from build123d import *

# Parameters (mm, degrees)
BOSS_EXTRUDE1_DEPTH  = 1.5875
M4_CLEARANCE_HOLE1_D = 4.5
BOSS_EXTRUDE2_DEPTH  = 3.175
FILLET1_R            = 3.5
M3_CLEARANCE_HOLE1_D = 3.4
SKETCH8_R            = 2.15
CUT_EXTRUDE1_DEPTH   = 4.1750001
SKETCH9_R            = 2.75
SKETCH9_R_2          = 2.15
BOSS_EXTRUDE3_DEPTH  = 0.75
SKETCH10_R           = 3.5
CUT_EXTRUDE2_DEPTH   = 2.5


with BuildPart() as part:
    # Sketch2 → Boss-Extrude1 (new body, symmetric)
    with BuildSketch(Plane.XY):
        with BuildLine():
            ThreePointArc((-17.942568571, -13.649816766), (-25.009816766, -13.417431429), (-24.777431429, -6.350183234))
            add(Edge.make_bspline(
                [(-24.777431429, -6.350183234), (-20.441430485, -2.271315687), (-12.829947979, 2.196277878), (-6.501150321, 4.42663028), (0, 5.19112324), (6.501150321, 4.42663028), (12.829947979, 2.196277878), (20.441430485, -2.271315687), (24.777431429, -6.350183234)],
                knots=[0, 0, 0, 0.1875, 0.3125, 0.4375, 0.5625, 0.6875, 0.8125, 1, 1, 1], degree=2))
            ThreePointArc((24.777431429, -6.350183234), (25.009816766, -13.417431429), (17.942568571, -13.649816766))
            add(Edge.make_bspline(
                [(-17.942568571, -13.649816766), (-14.268569515, -10.228684313), (-8.530052021, -6.883777878), (-4.178849679, -5.36413028), (0, -4.87862324), (4.178849679, -5.36413028), (8.530052021, -6.883777878), (14.268569515, -10.228684313), (17.942568571, -13.649816766)],
                knots=[0, 0, 0, 0.1875, 0.3125, 0.4375, 0.5625, 0.6875, 0.8125, 1, 1, 1], degree=2))
        make_face()
    extrude(amount=BOSS_EXTRUDE1_DEPTH, both=True)

    # M4 Clearance Hole1 (through all)
    with Locations(Plane.XY.offset(1.5875)):
        with Locations((21.36, -10), (0, 0)):
            Hole(M4_CLEARANCE_HOLE1_D / 2)

    # Sketch5 → Boss-Extrude2 (add)
    with BuildSketch(Plane(origin=(0, 0, -1.5875), x_dir=(-1, 0, 0), z_dir=(0, 0, -1))):
        with BuildLine():
            ThreePointArc((13.518770817, -20.368950039), (17.11, -26.460179221), (23.201229183, -22.868950039))
            Line((23.201229183, -22.868950039), (26.201229183, -11.25))
            ThreePointArc((26.201229183, -11.25), (22.61, -5.158770817), (16.518770817, -8.75))
            Line((16.518770817, -8.75), (13.518770817, -20.368950039))
        make_face()
    extrude(amount=-BOSS_EXTRUDE2_DEPTH)

    # Fillet1
    fillet1_edges = [part.edges().sort_by_distance(p)[0] for p in [
        (-15.752223744, -11.718824048, 0.7937488),
    ]]
    fillet(fillet1_edges, radius=FILLET1_R)

    # M3 Clearance Hole1 (through all)
    with Locations(Plane(origin=(0, 0, -1.5875), x_dir=(-1, 0, 0), z_dir=(0, 0, -1))):
        with Locations((18.36, -21.618950039)):
            Hole(M3_CLEARANCE_HOLE1_D / 2)

    # Sketch8 → Cut-Extrude1 (cut, through all)
    with BuildSketch(Plane(origin=(0, 0, -1.5875), x_dir=(-1, 0, 0), z_dir=(0, 0, -1))):
        with Locations((21.36, -10)):
            Circle(SKETCH8_R)
    extrude(amount=-CUT_EXTRUDE1_DEPTH, mode=Mode.SUBTRACT)

    # Sketch9 → Boss-Extrude3 (add)
    with BuildSketch(Plane(origin=(0, 0, -1.5875), x_dir=(-1, 0, 0), z_dir=(0, 0, -1))):
        with Locations((21.36, -10)):
            Circle(SKETCH9_R)
        with Locations((21.36, -10)):
            Circle(SKETCH9_R_2, mode=Mode.SUBTRACT)
    extrude(amount=BOSS_EXTRUDE3_DEPTH)

    # Sketch10 → Cut-Extrude2 (cut)
    with BuildSketch(Plane.XY.offset(1.5875)):
        with Locations((21.36, -10)):
            Circle(SKETCH10_R)
    extrude(amount=-CUT_EXTRUDE2_DEPTH, mode=Mode.SUBTRACT)


solid = part.part
Read the model definition and answer for the solid it produces. Units are mm, in the model's axes. A direction names the side the tool comes from. Round coordinates to 2 decimals unless told otherwise and drop trailing zeros. Loops run counter-clockwise (first coordinate to the right, second up) from the corner with the lowest first, then second, coordinate; pieces in that order, holes last. Notation, with made-up numbers: (28.25, -18.5) - (44.25, -18.5) arc R12 cw to (44.25, -1.5) - close; hole circle Ø9 at (23.25, 6.25). An arc over 180 degrees is marked (long way). One line per question, with ' | ' between items. Start each with the question number.
Q1. Find the intervals of material crossed by L1, parallel to Y at x = 0, z = 0.65; L2, parallel to Y at x = -19.5, z = -1.4; L3, parallel to X at y = -11.5, z = -0.8, in increasing order.
Q2. For a pull along X with two mould halves and no side action, classify faces 4 (the cylindrical face through (-23.9, -11.05, -1.96)), 5 (the flat face through (-23, -12, -2.338)), 6 (the cylindrical face through (-18.73, -23.28, 0.02)) as +X half, -X half, draft (parallel to the pull), parting line (faces both ways), or undercut.
Q3. For faces 1 (the flat face through (-14.362, -17.105, -0.022)), 2 (the flat face through (24, -10, -0.913)), 3 (the flat face through (-8, -6, 1.588)), determine the directions among +Z, -Z, +X, -X, +Y, -Y from which every point of the face is accessible in a straight line to the end or side of a thin tool.
Q4. Flat-ended cylindrical pins translate along their axes: pin 1 (5.5 mm diameter, centred on x = -18.36, y = -21.62, fed in from +Z); pin 2 (2 mm diameter, centred on x = -12, y = -7.5, fed in from -Z); pin 3 (2 mm diameter, centred on x = 23, y = -9.5, fed in from +Z). Find the tip coordinate at first contact, or state that the pin passes through.
Q5. Section A-A on y = -15.5 is taken. Give the vertices of the cut face in (x, z), plus the area to 3 significant figures.
Established:
1) L1: -5 to -2.25, 2.25 to 5 | L2: -26.49 to -22.88, -20.36 to -11.08, -8.92 to -1.97 | L3: -26.14 to -22.9, -19.82 to -14.93, 15.49 to 18.2, 24.52 to 26.13
2) face 4: parting line | face 5: draft | face 6: undercut
3) face 1: +Z, -Z | face 2: +Z | face 3: +Z, +X, -X, +Y, -Y
4) pin 1: z = 1.59 | pin 2: z = -1.59 | pin 3: z = -0.91
5) outline: (-25.1, -1.59) - (-14.78, -1.59) - (-14.78, 1.59) - (-25.1, 1.59) - close | area: 32.8 mm²
